from build123d import *

# Parameters (mm, degrees)
SKETCH1_R           = 9
SKETCH1_R_2         = 3
BOSS_EXTRUDE1_DEPTH = 10
BOSS_EXTRUDE3_DEPTH = 10
FILLET1_R           = 5
SKETCH6_R           = 2.5
CUT_EXTRUDE2_DEPTH  = 25


with BuildPart() as part:
    # Sketch1 → Boss-Extrude1 (new body)
    with BuildSketch(Plane(origin=(0, 0, 0), x_dir=(1, 0, 0), z_dir=(0, 1, 0))):
        with Locations(Location((0, 0, 0), (0, 0, 270))):
            Circle(SKETCH1_R)
        with Locations(Location((0, 0, 0), (0, 0, 270))):
            Circle(SKETCH1_R_2, mode=Mode.SUBTRACT)
    extrude(amount=BOSS_EXTRUDE1_DEPTH)

    # Sketch5 → Boss-Extrude3 (add)
    with BuildSketch(Plane.XZ):
        Polygon((7.933315826, 4.25), (24, 4.25), (24, 2.75), (7.137975048, 2.75), align=None)
        Polygon((7.137975048, -2.75), (7.933315826, -4.25), (24, -4.25), (24, -2.75), align=None)
    extrude(amount=-BOSS_EXTRUDE3_DEPTH)

    # Fillet1
    fillet1_edges = [part.edges().sort_by_distance(p)[0] for p in [
        (24, 0, -3.5),
        (24, 10, -3.5),
        (24, 10, 3.5),
        (24, 0, 3.5),
    ]]
    fillet(fillet1_edges, radius=FILLET1_R - 0.0001)  # a hair under: the kernel refuses the full size

    # Sketch6 → Cut-Extrude2 (cut)
    with BuildSketch(Plane.XY.offset(4.25)):
        with Locations((19, 5)):
            Circle(SKETCH6_R)
    extrude(amount=-CUT_EXTRUDE2_DEPTH, mode=Mode.SUBTRACT)


solid = part.part
Read the model definition and answer for the solid it produces. Units are mm, in the model's axes. A direction names the side the tool comes from. Give positions to 0.01 mm unless a question says otherwise; leave off trailing zeros. Write each loop counter-clockwise with the first axis right and the second up, starting at its lowest first coordinate (ties: lowest second). Pieces come first, ordered by that corner, then holes. Notation, with made-up numbers: (43, 30.25) - (80, 30.25) arc R20 cw to (80, 51.25) - close; hole circle Ø11 at (7.5, -22.5). An arc over 180 degrees is marked (long way). Answer in a Markdown table with one row per item. Add a question column.
Item 1: Find the intervals of material crossed by L1, parallel to Z at x = 16, y = 0.75; L2, parallel to Y at x = 19, z = -3.3; L3, parallel to X at y = 2.5, z = 0, in increasing order.
Item 2: Section C-C, the plane z = 0 is taken. Write down the section's boundary in (x, y), and give its area (3 significant figures).
Item 3: Section A-A, the plane x = 16 is taken. Write down the section's boundary in (y, z), and give its area (3 significant figures).
Item 4: A tool of negligible diameter and unlimited length cuts with its end or side. For faces 1 (the face through (15, 5, 2.75)), 2 (the face through (23, 2, -3)), 3 (the face through (14, 5, -4.25)), 4 (the face through (14, 5, 4.25)), 5 (the face through (22, 9, -3)), from which of +Z, -Z, +X, -X, +Y, -Y can it reach the whole face along a straight path? Write none if from no direction.
Item 5: Flat-ended cylindrical pins translate along their axes: P1, Ø1.5, axis at y = 2.5, z = -7, coming from the -X side; P2, Ø6, axis at x = 2, y = 3.5, coming from the -Z side; P3, Ø6, axis at x = 19, y = 5, coming from the -Z side. Find the tip coordinate at first contact, or state that the pin passes through.
Item 6: Section B-B, the plane y = 6.25 is taken. Write down the section's boundary in (x, z).
Item 7: Determine the mould class of faces 6 (the face through (16.5, 5.1, 3.5)), 7 (the face through (22, 1, 3)), 8 (the face through (16.5, 5.1, -3.5)), 9 (the face through (15, 5, -2.75)) for opening direction X: pulls with the +X half, pulls with the -X half, needs draft (parallel to the pull), parting line crosses it, or undercut.
Item 8: Section D-D, the plane y = 9 is taken. Write down the section's boundary in (x, z).
Recorded:
| question | item | result |
|---|---|---|
| 1 | L1 | z = -4.25 to -2.75, 2.75 to 4.25 |
| 1 | L2 | y = 0 to 2.5, 7.5 to 10 |
| 1 | L3 | x = -9 to -3, 3 to 9 |
| 2 | outline | (-9, 0) - (-3, 0) - (-3, 10) - (-9, 10) - close; (3, 0) - (9, 0) - (9, 10) - (3, 10) - close |
| 2 | area | 120 mm2 |
| 3 | outline | (0, -4.25) - (10, -4.25) - (10, -2.75) - (0, -2.75) - close; (0, 2.75) - (10, 2.75) - (10, 4.25) - (0, 4.25) - close |
| 3 | area | 30.0 mm2 |
| 4 | face 1 | +X, +Y, -Y |
| 4 | face 2 | +Z, -Z, +X, -Y |
| 4 | face 3 | -Z, +X, +Y, -Y |
| 4 | face 4 | +Z, +X, +Y, -Y |
| 4 | face 5 | +Z, -Z, +X, +Y |
| 5 | P1 | stops at x = -6.48 |
| 5 | P2 | stops at z = -9 |
| 5 | P3 | stops at z = -4.25 |
| 6 | outline | (7.93, -4.25) - (16.83, -4.25) - (16.83, -2.75) - (8.57, -2.75) arc R9 ccw to (8.57, 2.75) - (16.83, 2.75) - (16.83, 4.25) - (7.93, 4.25) arc R9 ccw (long way) to start; (21.17, -4.25) - (23.84, -4.25) - (23.84, -2.75) - (21.17, -2.75) - close; (21.17, 2.75) - (23.84, 2.75) - (23.84, 4.25) - (21.17, 4.25) - close; hole circle Ø6 at (0, 0) |
| 7 | face 6 | undercut |
| 7 | face 7 | pulls with the +X half |
| 7 | face 8 | undercut |
| 7 | face 9 | needs draft |
| 8 | outline | (7.93, -4.25) - (22, -4.25) - (22, -2.75) - (8.57, -2.75) arc R9 ccw to (8.57, 2.75) - (22, 2.75) - (22, 4.25) - (7.93, 4.25) arc R9 ccw (long way) to start; hole circle Ø6 at (0, 0) |
